Can you work these out from the model? Positions are in its coordinate system, mm. A direction names the side the tool comes from. Give positions to 0.01 mm unless a question says otherwise; leave off trailing zeros. Write each loop counter-clockwise with the first axis right and the second up, starting at its lowest first coordinate (ties: lowest second). Pieces come first, ordered by that corner, then holes. Notation, with made-up numbers: M 0.5,65.25 L 39.5,65.25 A23 cw 39.5,97.25 Z; hole C 78,85.25 d11. An arc over 180 degrees is marked long. Write each question's results on one line, items separated by ' | '.
from build123d import *

# Parameters (mm, degrees)
BOSS_EXTRUDE1_DEPTH = 10
BOSS_EXTRUDE2_DEPTH = 15
FILLET1_R           = 10
SKETCH3_W           = 120
SKETCH3_H           = 4
BOSS_EXTRUDE3_DEPTH = 15


with BuildPart() as part:
    # Sketch1 → Boss-Extrude1 (new body)
    with BuildSketch(Plane.XY):
        with BuildLine():
            ThreePointArc((-4.079215611, 5.75), (0, 7.05), (4.079215611, 5.75))
            Line((4.079215611, 5.75), (-4.079215611, 5.75))
        make_face()
        with BuildLine():
            Line((-4.079215611, 5.75), (4.079215611, 5.75))
            ThreePointArc((4.079215611, 5.75), (0, -7.05), (-4.079215611, 5.75))
        make_face()
        with BuildLine():
            ThreePointArc((-2.554236133, 1.756666667), (0, -3.1), (2.554236133, 1.756666667))
            ThreePointArc((2.554236133, 1.756666667), (0, 3.1), (-2.554236133, 1.756666667))
        make_face(mode=Mode.SUBTRACT)
    extrude(amount=BOSS_EXTRUDE1_DEPTH)

    # Sketch2 → Boss-Extrude2 (add)
    with BuildSketch(Plane(origin=(0, 0, 0), x_dir=(-1, 0, 0), z_dir=(0, 0, -1))):
        with BuildLine():
            Line((-60, -19.5), (60, -19.5))
            Line((60, -19.5), (60, -7))
            Line((60, -7), (12.5, -7))
            Line((12.5, -7), (12.5, 0))
            ThreePointArc((12.5, 0), (0, 12.5), (-12.5, 0))
            Line((-12.5, 0), (-12.5, -7))
            Line((-12.5, -7), (-60, -7))
            Line((-60, -7), (-60, -19.5))
        make_face()
    extrude(amount=BOSS_EXTRUDE2_DEPTH)

    # Fillet1
    fillet1_edges = [part.edges().sort_by_distance(p)[0] for p in [
        (-12.5, -7, -7.5),
        (12.5, -7, -7.5),
    ]]
    fillet(fillet1_edges, radius=FILLET1_R)

    # Sketch3 → Boss-Extrude3 (add)
    with BuildSketch(Plane.XY):
        with Locations((0, -17.5)):
            Rectangle(SKETCH3_W, SKETCH3_H)
    extrude(amount=BOSS_EXTRUDE3_DEPTH)


solid = part.part
Item 1: I want a section at D-D, the plane y = -8.5. Please give me the cut outline in (x, z).
Geometry says:
outline: M -60,-15 L 60,-15 L 60,0 L -60,0 Z
Item 2: I'm going to push flat-ended pins straight in: pin 1 (16.5 mm diameter, centred on x = 12.5, z = 11, fed in from +Y); pin 2 (12 mm diameter, centred on y = -4, z = 8.5, fed in from +X); pin 3 (7 mm diameter, centred on x = -2.5, y = 2, fed in from +Z). Where does each tip first touch, or does it pass through?
Geometry says:
pin 1: stops at y = 5.58 | pin 2: stops at x = 7.05 | pin 3: stops at z = 10
Item 3: If I drill on line 1 (Y direction, x = 0, z = 2.75); line 2 (Y direction, x = -1, z = 5); line 3 (X direction, y = 0, z = 6), over which ranges is the centre line in solid material (lowest first)? Write a range as from..to.
Geometry says:
line 1: y = -19.5..-15.5, -7.05..-3.1, 3.1..7.05 | line 2: y = -19.5..-15.5, -6.98..-2.93, 2.93..6.98 | line 3: x = -7.05..-3.1, 3.1..7.05
Item 4: Thinking about a two-plate mould opening in Y: for faces 6 (the face through (-0.251, 12.497, -7.395)), 7 (the face through (-1, -19.5, 0)), 8 (the face through (-1, -17, 15)), 9 (the face through (0, 0, 0)), which applies, +Y half, -Y half, draft (parallel to the pull), parting line (faces both ways), or undercut?
Geometry says:
face 6: +Y half | face 7: -Y half | face 8: draft | face 9: undercut
Item 5: For faces 1 (the face through (-60, -15, -4)), 2 (the face through (-41, -7, -7)), 3 (the face through (-1.5, -3, 10)), 4 (the face through (41, -7, -7)), 5 (the face through (1, -10, -15)), which set-ups out of +Z, -Z, +X, -X, +Y, -Y let a thin tool reach every point of the face, with its end or its side?
Geometry says:
face 1: +Z, -Z, -X, +Y, -Y | face 2: +Z, -Z, -X, +Y | face 3: +Z, +X, -X, +Y | face 4: +Z, -Z, +X, +Y | face 5: -Z, +X, -X, +Y, -Y
Item 6: I want a section at B-B, the plane x = 0. Please give me the cut outline in (y, z), and give its area (3 significant figures).
Geometry says:
outline: M -19.5,-15 L 12.5,-15 L 12.5,0 L 7.05,0 L 7.05,10 L 3.1,10 L 3.1,0 L -3.1,0 L -3.1,10 L -7.05,10 L -7.05,0 L -15.5,0 L -15.5,15 L -19.5,15 Z | area: 619 mm2
Item 7: I want a section at C-C, the plane z = 12. Please give me the cut outline in (x, y), and give its area (3 significant figures).
Geometry says:
outline: M -60,-19.5 L 60,-19.5 L 60,-15.5 L -60,-15.5 Z | area: 480 mm2
Item 8: I want a section at A-A, the plane z = 6.5. Please give me the cut outline in (x, y), and give its area (3 significant figures).
Geometry says:
outline: M -60,-19.5 L 60,-19.5 L 60,-15.5 L -60,-15.5 Z; C 0,0 d14.1; hole C 0,0 d6.2 | area: 606 mm2
